from build123d import *

# Parameters (mm, degrees)
BOSS_EXTRUDE1_DEPTH = 6.35
FILLET1_R           = 203.2
FILLET2_R           = 355.6
FILLET3_R           = 19.05
FILLET4_R           = 19.05
FILLET5_R           = 19.05
FILLET6_R           = 19.05
SKETCH2_R           = 14.2875
CUT_EXTRUDE1_DEPTH  = 6.35


with BuildPart() as part:
    # Sketch1 → Boss-Extrude1 (new body)
    with BuildSketch(Plane.XY):
        Polygon((0, 0), (215.9, 0), (215.9, 50.8), (0, 50.8), (-166.237074401, 1.544570548), (-152.4, -45.155555556), align=None)
    extrude(amount=BOSS_EXTRUDE1_DEPTH)

    # Fillet1
    fillet1_edges = [part.edges().sort_by_distance(p)[0] for p in [
        (0, 0, 3.175),
    ]]
    fillet(fillet1_edges, radius=FILLET1_R)

    # Fillet2
    fillet2_edges = [part.edges().sort_by_distance(p)[0] for p in [
        (0, 50.8, 3.175),
    ]]
    fillet(fillet2_edges, radius=FILLET2_R)

    # Fillet3
    fillet3_edges = [part.edges().sort_by_distance(p)[0] for p in [
        (-166.237074401, 1.544570548, 3.175),
    ]]
    fillet(fillet3_edges, radius=FILLET3_R)

    # Fillet4
    fillet4_edges = [part.edges().sort_by_distance(p)[0] for p in [
        (-152.4, -45.155555556, 3.175),
    ]]
    fillet(fillet4_edges, radius=FILLET4_R)

    # Fillet5
    fillet5_edges = [part.edges().sort_by_distance(p)[0] for p in [
        (215.9, 50.8, 3.175),
    ]]
    fillet(fillet5_edges, radius=FILLET5_R)

    # Fillet6
    fillet6_edges = [part.edges().sort_by_distance(p)[0] for p in [
        (215.9, 0, 3.175),
    ]]
    fillet(fillet6_edges, radius=FILLET6_R)

    # Sketch2 → Cut-Extrude1 (cut)
    with BuildSketch(Plane.XY.offset(6.35)):
        with Locations((-134.33022138, -14.825444286)):
            Circle(SKETCH2_R)
        with Locations((187.858901067, 25.448520628)):
            Circle(SKETCH2_R)
    extrude(amount=-CUT_EXTRUDE1_DEPTH, mode=Mode.SUBTRACT)


solid = part.part
Could you check a few things on this model? Use its own coordinates, in mm. Give positions to 0.01 mm unless a question says otherwise; leave off trailing zeros. Order: outer loops, then holes, each group sorted by start corner. A loop starts at its lowest first (then second) coordinate and runs counter-clockwise, first axis right, second up. Notation, with made-up numbers: (-10.75, 2) -> (14.25, 2) arc R11 cw to (14.25, 11) -> close; hole circle Ø6 at (68.5, 37). An arc over 180 degrees is marked (long way). Answer in a Markdown table with one row per item. Add a question column.
Item 1: Imagine slicing it at B-B (x = 88.5). List the corners of the cut face in (y, z) for me, and give its area (3 significant figures).
Item 2: We'd pull the mould along X, two halves only. Please class faces 1 (the flat face through (112, 0, 3)), 2 (the cylindrical face through (1.24, 47.22, 3.22)), 3 (the cylindrical face through (201.06, 19.98, 3.22)): pulls with the +X half, pulls with the -X half, needs draft (parallel to the pull), parting line crosses it, or undercut.
Item 3: Imagine slicing it at C-C (x = -4.5). List the corners of the cut face in (y, z) for me, and give its area (3 significant figures).
Item 4: Please list where these lines run through material, in increasing order: probe 1 along Y at (x, z) = (86.5, 1); probe 2 along X at (y, z) = (2, 2.25); probe 3 along Y at (x, z) = (6.5, 3.5).
Item 5: I'm going to push a flat-ended pin straight in: P1, Ø3, axis at x = 79.5, z = 2.5, coming from the -Y side. Where does the tip first touch, or does it pass through?
Item 6: Imagine slicing it at A-A (z = 3). Count the separate pieces of the cut face and the enclosed holes in it, and give its area (3 significant figures).
Result:
| question | item | result |
|---|---|---|
| 1 | outline | (0, 0) -> (50.8, 0) -> (50.8, 6.35) -> (0, 6.35) -> close |
| 1 | area | 323 mm2 |
| 2 | face 1 | needs draft |
| 2 | face 2 | pulls with the -X half |
| 2 | face 3 | undercut |
| 3 | outline | (-2.86, 0) -> (46.35, 0) -> (46.35, 6.35) -> (-2.86, 6.35) -> close |
| 3 | area | 312 mm2 |
| 4 | probe 1 | 0 to 50.8 |
| 4 | probe 2 | -156.19 to 205.35 |
| 4 | probe 3 | -1.3 to 47.93 |
| 5 | P1 | y = 0 |
| 6 | separate pieces | 1 |
| 6 | enclosed holes | 2 |
| 6 | area | 17,400 mm2 |
